Source: CAD feature listing. Evaluate the final solid. Frame: model axes, mm. A direction names the side the tool comes from. Round coordinates to 2 decimals unless told otherwise and drop trailing zeros. Order: outer loops, then holes, each group sorted by start corner. A loop starts at its lowest first (then second) coordinate and runs counter-clockwise, first axis right, second up. Notation, with made-up numbers: (33, 47.5) - (44, 47.5) arc R28 ccw to (44, 75.5) - close; hole circle Ø2 at (53, 32.25). An arc over 180 degrees is marked (long way). Put each result on its own line as item: value. Start each with the question number.
1) Access query for faces 1 (the face through (14.668, -20, 10)), 2 (the face through (-14.668, -20, 10)), 3 (the face through (-1, 70.556, 3)). Directions: +Z, -Z, +X, -X, +Y, -Y. A direction counts if a zero-diameter tool reaches every point of the face in a straight line with its end or side. Return the directions, or none.
2) Section D-D on x = 43.5. Output: boundary loops of the cut face in (y, z), then the cut area to 3 significant figures.
3) Section A-A on z = 14. Output: boundary loops of the cut face in (x, y), then the cut area to 3 significant figures.
4) Line query: probe 1 along Z at (x, y) = (29, -17.5); probe 2 along Y at (x, z) = (8, 25); probe 3 along Y at (x, z) = (-0.5, 17) (3 decimals). Output: solid intervals per line, ascending. Write a range as [from, to].
5) Contact query for a flat-ended pin moving along its axis: P1, Ø1.5, axis at x = 16.5, z = 26, coming from the -Y side. Output: stop coordinate, or through.
6) Section B-B on y = -21.5. Output: boundary loops of the cut face in (x, z).
```python
from build123d import *

# Parameters (mm, degrees)
F0_W     = 152.4
F0_H     = 141.1111171471
F1_DEPTH = 6.35
F2_W     = 14.6685
F2_H     = 50.8
F3_DEPTH = 25.4
F4_R     = 25.39999
F6_DEPTH = 76.2


# Not quite as in the source:
# - a fillet or chamfer is up to 0.001 mm smaller than in the source, because OpenCascade refuses the exact size


with BuildPart() as f1:
    # F0 (on Top) → F1 (new body)
    with BuildSketch(Plane.XY):
        Rectangle(F0_W, F0_H)
    extrude(amount=F1_DEPTH)

    # F2 (on face) → F3 (join)
    with BuildSketch(Plane.XY.offset(6.35)):
        with Locations((-7.33425, -19.7555585735)):
            Rectangle(F2_W, F2_H)
        with Locations((7.33425, -19.7555585735)):
            Rectangle(F2_W, F2_H)
    extrude(amount=F3_DEPTH)

    # F4 (radius 25.4 in the source; OpenCascade refuses exactly that, so slightly less here)
    f4_edges = [f1.edges().sort_by_distance(p)[0] for p in [
        (0, 5.644441, 31.75),
        (0, -45.155559, 31.75),
    ]]
    fillet(f4_edges, radius=F4_R)

    # F5 (on face) → F6 (cut)
    with BuildSketch(Plane(origin=(-14.6685, 0, 0), x_dir=(0, -1, 0), z_dir=(-1, 0, 0))):
        with BuildLine():
            Line((19.7555585735, 11.557), (19.7555585735, 27.432))
            ThreePointArc((19.7555585735, 27.432), (11.8180585735, 19.4945), (19.7555585735, 11.557))
        make_face()
        with BuildLine():
            ThreePointArc((27.6930585735, 19.4945), (25.3682186492, 25.1071600757), (19.7555585735, 27.432))
            Line((19.7555585735, 27.432), (19.7555585735, 11.557))
            ThreePointArc((19.7555585735, 11.557), (25.3682186492, 13.8818399243), (27.6930585735, 19.4945))
        make_face()
    extrude(amount=-F6_DEPTH, mode=Mode.SUBTRACT)


solid = f1.part
```
Answer sheet:
1. face 1: +Z, +X, +Y, -Y
1. face 2: +Z, -X, +Y, -Y
1. face 3: +Z, -Z, +X, -X, +Y
2. outline: (-70.56, 0) - (70.56, 0) - (70.56, 6.35) - (-70.56, 6.35) - close
2. area: 896 mm^2
3. outline: (-14.67, -43.98) - (14.67, -43.98) - (14.67, -25.48) - (-14.67, -25.48) - close; (-14.67, -14.03) - (14.67, -14.03) - (14.67, 4.47) - (-14.67, 4.47) - close
3. area: 1,090 mm^2
4. probe 1: [0, 6.35]
4. probe 2: [-37, -25.47], [-14.04, -2.51]
4. probe 3: [-42.815, -27.291], [-12.22, 3.304]
5. P1: through
6. outline: (-76.2, 0) - (76.2, 0) - (76.2, 6.35) - (14.67, 6.35) - (14.67, 11.75) - (-14.67, 11.75) - (-14.67, 6.35) - (-76.2, 6.35) - close; (-14.67, 27.24) - (14.67, 27.24) - (14.67, 31.69) - (-14.67, 31.69) - close
